from build123d import *

# Parameters (mm, degrees)
MODEL_R             = 1.2
MODEL_W             = 5.35
MODEL_H             = 11
MODEL_W_2           = 9
MODEL_H_2           = 5.35
BOSS_EXTRUDE1_DEPTH = 5.35


with BuildPart() as part:
    # Model → Boss-Extrude1 (new body)
    with BuildSketch(Plane.XY):
        with BuildLine():
            Line((58.85, 269), (33, 269))
            ThreePointArc((33, 269), (25.928932188, 266.071067812), (23, 259))
            Line((23, 259), (23, 150))
            ThreePointArc((23, 150), (20.071067812, 142.928932188), (13, 140))
            Line((13, 140), (10, 140))
            ThreePointArc((10, 140), (2.928932188, 137.071067812), (0, 130))
            Line((0, 130), (0, 10))
            ThreePointArc((0, 10), (2.928932188, 2.928932188), (10, 0))
            Line((10, 0), (58.85, 0))
            Line((58.85, 0), (58.85, 45))
            Line((58.85, 45), (64.2, 45))
            Line((64.2, 45), (64.2, 74.666666667))
            Line((64.2, 74.666666667), (58.85, 74.666666667))
            Line((58.85, 74.666666667), (58.85, 119.666666667))
            Line((58.85, 119.666666667), (64.2, 119.666666667))
            Line((64.2, 119.666666667), (64.2, 149.333333333))
            Line((64.2, 149.333333333), (58.85, 149.333333333))
            Line((58.85, 149.333333333), (58.85, 194.333333333))
            Line((58.85, 194.333333333), (64.2, 194.333333333))
            Line((64.2, 194.333333333), (64.2, 224))
            Line((64.2, 224), (58.85, 224))
            Line((58.85, 224), (58.85, 269))
        make_face()
        with Locations((2.5, 88.027872499)):
            Circle(MODEL_R, mode=Mode.SUBTRACT)
        with Locations((44.6, 37.227872499)):
            Circle(MODEL_R, mode=Mode.SUBTRACT)
        with Locations((16.7, 37.227872499)):
            Circle(MODEL_R, mode=Mode.SUBTRACT)
        with Locations((50.5, 89.327872499)):
            Circle(MODEL_R, mode=Mode.SUBTRACT)
        with Locations((29.175, 160)):
            Rectangle(MODEL_W, MODEL_H, mode=Mode.SUBTRACT)
        with Locations((45.35, 131.325)):
            Rectangle(MODEL_W_2, MODEL_H_2, mode=Mode.SUBTRACT)
        with Locations((29.175, 121)):
            Rectangle(MODEL_W, MODEL_H, mode=Mode.SUBTRACT)
        with Locations((45.35, 41.675)):
            Rectangle(MODEL_W_2, MODEL_H_2, mode=Mode.SUBTRACT)
        with Locations((29.175, 52)):
            Rectangle(MODEL_W, MODEL_H, mode=Mode.SUBTRACT)
        with Locations((29.175, 13)):
            Rectangle(MODEL_W, MODEL_H, mode=Mode.SUBTRACT)
        with BuildLine():
            Line((5, 123.711859862), (13, 123.711859862))
            ThreePointArc((13, 123.711859862), (13.707106781, 124.004753081), (14, 124.711859862))
            Line((14, 124.711859862), (14, 131.711859862))
            ThreePointArc((14, 131.711859862), (13.707106781, 132.418966643), (13, 132.711859862))
            Line((13, 132.711859862), (5, 132.711859862))
            ThreePointArc((5, 132.711859862), (4.292893219, 132.418966643), (4, 131.711859862))
            Line((4, 131.711859862), (4, 124.711859862))
            ThreePointArc((4, 124.711859862), (4.292893219, 124.004753081), (5, 123.711859862))
        make_face(mode=Mode.SUBTRACT)
    extrude(amount=BOSS_EXTRUDE1_DEPTH)


solid = part.part
Can you work these out from the model? Positions are in its coordinate system, mm. A direction names the side the tool comes from. Give positions to 0.01 mm unless a question says otherwise; leave off trailing zeros. Loops run counter-clockwise (first coordinate to the right, second up) from the corner with the lowest first, then second, coordinate; pieces in that order, holes last. Notation, with made-up numbers: (20.25, 52.25) - (30.25, 52.25) arc R23 cw to (30.25, 77.25) - close; hole circle Ø8 at (32.5, 78). An arc over 180 degrees is marked (long way). One line per item, written item: value.
(1) If we mould it in two halves opening along Y, with no side actions, what happens to faces 1 (the face through (49.85, 131, 3)), 2 (the face through (26.01, 266.15, 2.64)), 3 (the face through (29, 154.5, 3)), 4 (the face through (64.2, 60, 3))? For each: released by +Y, released by -Y, zero draft, split by the parting line, or undercut.
Verdict:
face 1: undercut
face 2: released by +Y
face 3: undercut
face 4: zero draft
(2) I need wall thicknesses on line 1 along Y through (x, z) = (50.5, 2.4); line 2 along Y through (x, z) = (9.5, 3); line 3 along X through (y, z) = (87, 3.25). Which ranges of each line are inside material? Lowest first, please.
Verdict:
line 1: 0 to 88.13, 90.53 to 269
line 2: 0.01 to 123.71, 132.71 to 139.99
line 3: 0 to 1.88, 3.12 to 58.85
(3) If we section it at A-A, the plane y = 179.5: List the corners of the cut face in (x, z) for me, plus the area to 3 significant figures.
Verdict:
outline: (23, 0) - (58.85, 0) - (58.85, 5.35) - (23, 5.35) - close
area: 192 mm^2
(4) I'm going to push flat-ended pins straight in: pin 1 (2.5 mm diameter, centred on y = 162, z = 1.5, fed in from +X); pin 2 (1.6 mm diameter, centred on x = 29, z = 3, fed in from +Y); pin 3 (1.9 mm diameter, centred on x = 44.6, y = 37.23, fed in from -Z); pin 4 (2.5 mm diameter, centred on x = 61, z = 1.5, fed in from +Y). Where does each tip first touch, or does it pass through?
Verdict:
pin 1: x = 58.85
pin 2: y = 268.47
pin 3: through
pin 4: y = 224
(5) On a 3-axis mill with a long thin cutter (end or side, diameter ignored), from which of +Z, -Z, +X, -X, +Y, -Y can I reach the whole of each face in a straight line? I mean faces 5 (the face through (14, 128, 3)), 6 (the face through (62, 74.667, 3)), 7 (the face through (58.85, 22, 3)). Say none if no direction works.
Verdict:
face 5: +Z, -Z
face 6: +Z, -Z, +X
face 7: +Z, -Z, +X, -Y
(6) If we section it at C-C, the plane y = 78: List the corners of the cut face in (x, z) for me.
Verdict:
outline: (0, 0) - (58.85, 0) - (58.85, 5.35) - (0, 5.35) - close
(7) If we section it at B-B, the plane z = 0.85: State how many separate pieces and enclosed holes the cut face has, plus the area to 3 significant figures.
Verdict:
separate pieces: 1
enclosed holes: 11
area: 12,900 mm^2
